Could you check a few things on this model? Use its own coordinates, in mm. Face numbers are marked on the shaded views. A direction names the side the tool comes from. Coordinates: 2 decimals unless noted, no trailing zeros. Loops run counter-clockwise (first coordinate to the right, second up) from the corner with the lowest first, then second, coordinate; pieces in that order, holes last. Notation, with made-up numbers: (5.5, -31) - (33.5, -31) arc R22 cw to (33.5, -18) - close; hole circle Ø11 at (34.25, -25.5). An arc over 180 degrees is marked (long way). Put each result on its own line as item: value. Start each with the question number.
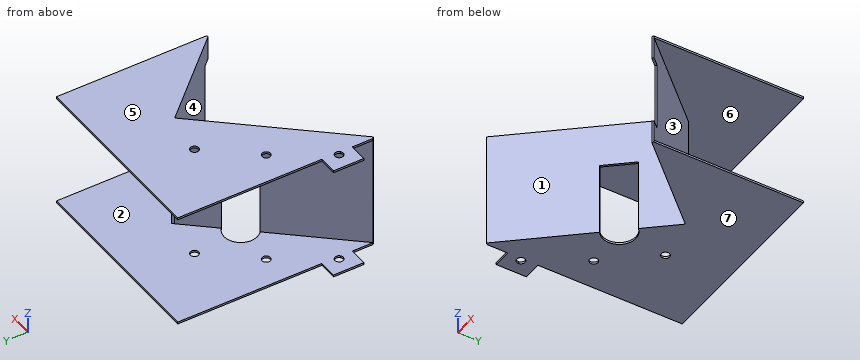
```python
from build123d import *
from build123d.topology import SkipClean

# Parameters (mm, degrees)
BOSS_EXTRUDE1_DEPTH    = 177.8
SKETCH2_R              = 6.35
BOSS_EXTRUDE2_DEPTH    = 3.175
CUT_EXTRUDE1_START     = -3.175
CUT_EXTRUDE1_OUTLINE_W = 50.8
CUT_EXTRUDE1_OUTLINE_H = 108.585
CUT_EXTRUDE1_DEPTH     = 3.175
SKETCH4_R              = 25.4
CUT_EXTRUDE2_DEPTH     = 5.08
BOSS_EXTRUDE3_DEPTH    = 3.175
BOSS_EXTRUDE4_START    = -3.175
BOSS_EXTRUDE4_DEPTH    = 3.175
SKETCH2_3_R            = 6.35
CUT_EXTRUDE3_DEPTH     = 203.2
SKETCH7_W              = 105.41
SKETCH7_H              = 15.24
CUT_EXTRUDE4_DEPTH     = 3.175


# Read off the part's stored shape, not the designer's step: Cut-Extrude1
with BuildPart() as part:
    # Sketch1 → Boss-Extrude1 (new body)
    with BuildSketch(Plane.XY):
        Polygon((174.215968213, 205.236242664), (176.61217113, 203.153255247), (6.420733494, 7.37040221), (4.024530577, 9.453389627), align=None)
        Polygon((176.61217113, 203.153255247), (176.61217113, 207.680393207), (174.215968213, 205.236242664), align=None)
        Polygon((176.61217113, 203.153255247), (176.61217113, 207.680393207), (294.86623267, 79.97762329), (292.609334988, 77.887713122), align=None)
    extrude(amount=BOSS_EXTRUDE1_DEPTH)

    # Sketch2 → Boss-Extrude2 (add)
    with BuildSketch(Plane(origin=(0, 0, 0), x_dir=(-1, 0, 0), z_dir=(0, 0, -1))):
        Polygon((-176.61217113, 207.680393207), (-294.86623267, 79.97762329), (-294.86623267, 308.57762329), (-4.03623267, 308.57762329), (-4.03623267, 9.466851346), align=None)
        with Locations((-109.551832016, 215.6073789)):
            Circle(SKETCH2_R, mode=Mode.SUBTRACT)
        with Locations((-50.099162461, 143.63835786)):
            Circle(SKETCH2_R, mode=Mode.SUBTRACT)
    boss_extrude2 = extrude(amount=-BOSS_EXTRUDE2_DEPTH)

    # Mirror1: Boss-Extrude2 across plane
    add(boss_extrude2.mirror(Plane.XY.offset(88.9)))

    # Cut-Extrude1 outline → Cut-Extrude1 (cut)
    with BuildSketch(Plane(origin=(-2.388376456, 2.076183978, 0), x_dir=(0.6560590289905027, 0.754709580222776, 0), z_dir=(-0.754709580222776, 0.6560590289905027, 0)).offset(CUT_EXTRUDE1_START)):
        with Locations((182.49489334, -57.4675)):
            Rectangle(CUT_EXTRUDE1_OUTLINE_W, CUT_EXTRUDE1_OUTLINE_H)
    extrude(amount=CUT_EXTRUDE1_DEPTH, mode=Mode.SUBTRACT)

    # Sketch4 → Cut-Extrude2 (cut)
    with BuildSketch(Plane.XY.offset(3.175)):
        with Locations((117.470149606, 139.752328242)):
            Circle(SKETCH4_R)
    extrude(amount=-CUT_EXTRUDE2_DEPTH, mode=Mode.SUBTRACT)

    # Sketch5 → Boss-Extrude3 (add)
    with BuildSketch(Plane(origin=(0, 0, 0), x_dir=(-1, 0, 0), z_dir=(0, 0, -1))):
        with BuildLine():
            Line((23.718677813, 87.809342908), (-4.03623267, 87.809342908))
            Line((-4.03623267, 87.809342908), (-4.03623267, 68.97229904))
            ThreePointArc((-4.03623267, 68.97229904), (2.710389506, 69.812621892), (6.35, 64.070123417))
            ThreePointArc((6.35, 64.070123417), (2.710389506, 58.327624943), (-4.03623267, 59.167947795))
            Line((-4.03623267, 59.167947795), (-4.03623267, 41.258157594))
            Line((-4.03623267, 41.258157594), (23.718677813, 41.258157594))
            Line((23.718677813, 41.258157594), (23.718677813, 87.809342908))
        make_face()
    extrude(amount=-BOSS_EXTRUDE3_DEPTH)

    # Sketch6 → Boss-Extrude4 (add)
    with BuildSketch(Plane.XY.offset(177.8).offset(BOSS_EXTRUDE4_START)):
        with BuildLine():
            Line((4.03623267, 68.97229904), (4.03623267, 87.809342908))
            Line((4.03623267, 87.809342908), (-23.718677813, 87.809342908))
            Line((-23.718677813, 87.809342908), (-23.718677813, 41.258157594))
            Line((-23.718677813, 41.258157594), (4.03623267, 41.258157594))
            Line((4.03623267, 41.258157594), (4.03623267, 59.167947795))
            ThreePointArc((4.03623267, 59.167947795), (-6.35, 64.070123417), (4.03623267, 68.97229904))
        make_face()
    extrude(amount=BOSS_EXTRUDE4_DEPTH)

    # Sketch2<3> → Cut-Extrude3 (cut)
    with SkipClean():  # the faces are left unmerged after this step: merging them gives an invalid solid
        with BuildSketch(Plane(origin=(0, 0, 0), x_dir=(-1, 0, 0), z_dir=(0, 0, -1))):
            with Locations((0, 64.070123417)):
                Circle(SKETCH2_3_R)
        extrude(amount=-CUT_EXTRUDE3_DEPTH, mode=Mode.SUBTRACT)

    # Sketch7 → Cut-Extrude4 (cut)
    with SkipClean():  # the faces are left unmerged after this step: merging them gives an invalid solid
        with BuildSketch(Plane(origin=(198.614996443, 183.919503291, 0), x_dir=(0, 0, -1), z_dir=(0.7337298645028701, 0.6794413042615234, 0))):
            with Locations((-88.265, -134.042327008)):
                Rectangle(SKETCH7_W, SKETCH7_H)
        extrude(amount=-CUT_EXTRUDE4_DEPTH, mode=Mode.SUBTRACT)


solid = part.part
```
(1) For pin 1 Ø8 at (x, z) = (185.5, 112) entering from +Y; pin 2 Ø5 at (x, z) = (86, 95.5) entering from -Y; pin 3 Ø8 at (x, z) = (211.5, 48.5) entering from -Y; pin 4 Ø11.5 at (x, y) = (50.1, 143.64) entering from -Z, each with a flat end and sliding along its axis, tell me the tip position at first contact or that it passes through.
(2) If we mould it in two halves opening along Z, with no side actions, what happens to the marked faces 4, 5, 6 and 7? For each: pulls with the +Z half, pulls with the -Z half, needs draft (parallel to the pull), parting line crosses it, or undercut.
(3) I want a section at A-A on z = 22.5. List the corners of the cut face in (x, y) for me.
(4) I want a section at B-B on x = 0. List the corners of the cut face in (y, z) for me (3 decimals).
(5) Which directions (+Z, -Z, +X, -X, +Y, -Y) give clear straight access to the entire face, cutting with the end or side of a thin tool? Please do the marked faces 1, 2 and 3.
(6) I want a section at C-C on y = 84. List the corners of the cut face in (x, z) for me (3 decimals), and give its area (3 significant figures).
(7) I need wall thicknesses on L1, parallel to Z at x = 232.5, y = 261.5 (3 decimals); L2, parallel to X at y = 123, z = 165; L3, parallel to X at y = 108, z = 153. Which ranges of each line are inside material? Lowest first, please. Write a range as [from, to].
(8) I want a section at D-D on z = 133. List the corners of the cut face in (x, y) for me.
Answer sheet:
1. pin 1: stops at y = 202.4
1. pin 2: stops at y = 96.04
1. pin 3: stops at y = 161.16
1. pin 4: passes through
2. face 4: needs draft
2. face 5: pulls with the +Z half
2. face 6: undercut
2. face 7: pulls with the -Z half
3. outline: (4.02, 9.45) - (6.42, 7.37) - (103.07, 118.55) - (100.68, 120.64) - close; (134, 158.98) - (136.4, 156.89) - (176.61, 203.15) - (292.61, 77.89) - (294.87, 79.98) - (176.61, 207.68) - (174.22, 205.24) - close
4. outline: (41.258, 0) - (57.72, 0) - (57.72, 3.175) - (41.258, 3.175) - close; (41.258, 174.625) - (57.72, 174.625) - (57.72, 177.8) - (41.258, 177.8) - close; (70.42, 0) - (87.809, 0) - (87.809, 3.175) - (70.42, 3.175) - close; (70.42, 174.625) - (87.809, 174.625) - (87.809, 177.8) - (70.42, 177.8) - close
5. face 1: +Z, -Z, -Y
5. face 2: +Y
5. face 3: +X, +Y
6. outline: (-23.719, 0) - (73.034, 0) - (73.034, 177.8) - (-23.719, 177.8) - (-23.719, 174.625) - (68.827, 174.625) - (68.827, 3.175) - (-23.719, 3.175) - close; (286.949, 0) - (294.866, 0) - (294.866, 3.175) - (291.141, 3.175) - (291.141, 35.56) - (286.949, 35.56) - close; (286.949, 140.97) - (291.141, 140.97) - (291.141, 174.625) - (294.866, 174.625) - (294.866, 177.8) - (286.949, 177.8) - close
6. area: 1,660 mm^2
7. L1: z = [0, 3.175], [174.625, 177.8]
7. L2: x = [102.73, 106.94], [250.83, 255.03]
7. L3: x = [89.69, 93.9], [264.73, 268.92]
8. outline: (4.02, 9.45) - (6.42, 7.37) - (176.61, 203.15) - (282.25, 89.07) - (284.51, 91.16) - (176.61, 207.68) - (174.22, 205.24) - close
